from build123d import *

# Parameters (mm, degrees)
CROQUIS2_R              = 2.975
CROQUIS2_R_2            = 2.5
SALIENTE_EXTRUIR1_DEPTH = 5
SALIENTE_EXTRUIR2_DEPTH = 21


with BuildPart() as part:
    # Croquis2 → Saliente-Extruir1 (new body)
    with BuildSketch(Plane(origin=(0, 0, 0), x_dir=(1, 0, 0), z_dir=(0, 1, 0))):
        with BuildLine():
            Line((-19.5, 6.523737612), (19.5, 6.523737612))
            ThreePointArc((19.5, 6.523737612), (26.023737612, 0), (19.5, -6.523737612))
            Line((19.5, -6.523737612), (-19.5, -6.523737612))
            ThreePointArc((-19.5, -6.523737612), (-26.023737612, 0), (-19.5, 6.523737612))
        make_face()
        with Locations(Location((0, 0, 0), (0, 0, 270))):
            Circle(CROQUIS2_R, mode=Mode.SUBTRACT)
        with Locations(Location((19.5, 0, 0), (0, 0, 270))):
            Circle(CROQUIS2_R_2, mode=Mode.SUBTRACT)
        with Locations(Location((-19.5, 0, 0), (0, 0, 270))):
            Circle(CROQUIS2_R_2, mode=Mode.SUBTRACT)
    extrude(amount=SALIENTE_EXTRUIR1_DEPTH)

    # Croquis2_4 → Saliente-Extruir2 (add)
    with BuildSketch(Plane(origin=(0, 0, 0), x_dir=(1, 0, 0), z_dir=(0, 1, 0))):
        with BuildLine():
            ThreePointArc((2.975, 0), (0, 2.975), (-2.975, 0))
            Line((-2.975, 0), (2.975, 0))
        make_face()
        with BuildLine():
            Line((2.975, 0), (-2.975, 0))
            ThreePointArc((-2.975, 0), (0, -2.975), (2.975, 0))
        make_face()
    extrude(amount=SALIENTE_EXTRUIR2_DEPTH)


solid = part.part
Geometry: final body of the model. Coordinates: model frame, mm. Give positions to 0.01 mm unless a question says otherwise; leave off trailing zeros. Loops run counter-clockwise (first coordinate to the right, second up) from the corner with the lowest first, then second, coordinate; pieces in that order, holes last. Notation, with made-up numbers: M 74.5,72.25 L 97.5,72.25 A37 ccw 97.5,108.25 Z; hole C 17,28 d11. An arc over 180 degrees is marked long. Put each result on its own line as item: value. Start each with the question number.
1) Cut plane D-D (x = -11.5). Output: boundary loops of the cut face in (y, z), then the cut area to 3 significant figures.
2) Cut plane B-B (x = 0). Output: boundary loops of the cut face in (y, z) (3 decimals).
3) Ray query, line 1 along X through (y, z) = (3.75, 0); line 2 along X through (y, z) = (2, 2); line 3 along Y through (x, z) = (-13.5, -5). Return the intervals inside material, ascending.
4) Cut plane C-C (y = 14). Output: boundary loops of the cut face in (x, z) (3 decimals), then the cut area to 3 significant figures.
5) Cut plane A-A (z = 0). Output: boundary loops of the cut face in (x, y) (3 decimals).
6) Pull-direction query (Z, two-part tool) for faces 1 (the cylindrical face through (-17, 2, 0)), 2 (the flat face through (0, 2, -6.524)), 3 (the cylindrical face through (-2.84, 12.89, 0.89)), 4 (the flat face through (0, 5, -4)); classes: pulls with the +Z half, pulls with the -Z half, needs draft (parallel to the pull), parting line crosses it, or undercut.
7) Contact query for flat-ended pins moving along their axis: pin 1 (1.5 mm diameter, centred on y = 18.5, z = -0.5, fed in from +X) (3 decimals); pin 2 (10 mm diameter, centred on x = -10.5, y = 17, fed in from +Z); pin 3 (4 mm diameter, centred on y = 2.5, z = 3.5, fed in from -X); pin 4 (1.5 mm diameter, centred on x = -6, z = 0.5, fed in from +Y). Output: stop coordinate, or through.
Verdict:
1. outline: M 0,-6.52 L 5,-6.52 L 5,6.52 L 0,6.52 Z
1. area: 65.2 mm2
2. outline: M 0,-6.524 L 5,-6.524 L 5,-2.975 L 21,-2.975 L 21,2.975 L 5,2.975 L 5,6.524 L 0,6.524 Z
3. line 1: -26.02 to -22, -17 to 17, 22 to 26.02
3. line 2: -25.71 to -21, -18 to 18, 21 to 25.71
3. line 3: 0 to 5
4. outline: C 0,0 d5.95
4. area: 27.8 mm2
5. outline: M -26.024,0 L -22,0 L -22,5 L -26.024,5 Z; M -17,0 L 17,0 L 17,5 L 2.975,5 L 2.975,21 L -2.975,21 L -2.975,5 L -17,5 Z; M 22,0 L 26.024,0 L 26.024,5 L 22,5 Z
6. face 1: undercut
6. face 2: pulls with the -Z half
6. face 3: parting line crosses it
6. face 4: needs draft
7. pin 1: x = 2.975
7. pin 2: through
7. pin 3: x = -25.85
7. pin 4: y = 5
